The model under review builds one solid part; all positions refer to its coordinate system, in mm. Round coordinates to 2 decimals unless told otherwise and drop trailing zeros. Order: outer loops, then holes, each group sorted by start corner. A loop starts at its lowest first (then second) coordinate and runs counter-clockwise, first axis right, second up. Notation, with made-up numbers: M 2.25,-5.75 L 43.25,-5.75 A18 cw 43.25,20.25 Z; hole C -8.75,26 d2. An arc over 180 degrees is marked long. Answer as a JSON object with one key per item and string values. Group by question number.
1. Mouldability with a two-part tool opening along X and no side actions: class faces 1 (the face through (6.988, -4.115, 2.083)), 2 (the face through (0.507, 4.674, 4.365)), 3 (the face through (6.4, -3.7, 0)), 4 (the face through (12.34, 4.56, 8.71)) as released by +X, released by -X, zero draft, split by the parting line, or undercut.
2. Add section B-B on x = 11.75. State the section outline as (y, z) points, and give its area (3 significant figures).
3. Clearance check with flat-ended pins moving along their axes: P1, Ø4.5, axis at x = 6.5, y = -7.83, coming from the -Z side; P2, Ø6, axis at x = 11, y = -0.5, coming from the +Z side. State where each tip first meets the part, or that it passes through.
4. Add section A-A on z = 7.5. State the section outline as (x, y) points.
5. To check wall thickness, follow probe 1 along Y at (x, z) = (6.5, 2.6); probe 2 along Y at (x, z) = (4, 1); probe 3 along X at (y, z) = (-7.75, 4). State the ranges of each line that lie inside material, in increasing order. Write a range as [from, to].
```python
from build123d import *

# Parameters (mm, degrees)
RESSALTO_EXTRUS_O1_DEPTH = 13
ESBO_O3_R                = 3.75
CORTE_EXTRUS_O1_DEPTH    = 15
FILETE1_R                = 0.5


with BuildPart() as part:
    # Esboço2 → Ressalto-extrusão1 (new body)
    with BuildSketch(Plane(origin=(0, 0, 0), x_dir=(0, 0, -1), z_dir=(1, 0, 0))):
        Polygon((0, 5.167385512), (0, -18.032614488), (-9.609754647, 5.167385512), align=None)
    extrude(amount=RESSALTO_EXTRUS_O1_DEPTH)

    # Esboço3 → Corte-extrusão1 (cut)
    with BuildSketch(Plane(origin=(0, 0, 0), x_dir=(-1, 0, 0), z_dir=(0, 0, -1))):
        with Locations((-6.5, -7.832614488)):
            Circle(ESBO_O3_R)
    extrude(amount=-CORTE_EXTRUS_O1_DEPTH, mode=Mode.SUBTRACT)

    # Chanfro1
    # the kernel refuses this chamfer: 1, 0.765366865 mm, written as the material it takes off along each edge
    with BuildSketch(Plane(origin=(12.333333333, 4.598349918, 8.679921653), x_dir=(0.6671683756339832, -0.6671683756339838, -0.3313196600080107), z_dir=(0.7268306825413349, 0.4856527354584224, 0.485652735458423))) as chanfro1_piece_1:
        Polygon((-0.578784303, 0.323797402), (0.920087701, 0.323797402), (-0.341303398, -0.647594805), align=None)
    extrude(amount=1.33373176, mode=Mode.SUBTRACT)
    with BuildSketch(Plane(origin=(0.666666667, 4.598349918, 8.679921653), x_dir=(-0.6671683756339831, -0.6671683756339838, -0.3313196600080107), z_dir=(-0.7268306825413349, 0.48565273545842236, 0.485652735458423))) as chanfro1_piece_2:
        Polygon((-0.578784303, -0.323797402), (0.920087701, -0.323797402), (-0.341303398, 0.647594805), align=None)
    extrude(amount=1.33373176, mode=Mode.SUBTRACT)
    with BuildSketch(Plane(origin=(13, 5.167385512, 12.181437635), x_dir=(-0.9996219169112968, 0.02749587661058651, 0), z_dir=(0, 0, -1))) as chanfro1_piece_3:
        with BuildLine():
            Line((1.028673195, 0), (-0.056547155, -1.027117794))
            Line((-0.056547155, -1.027117794), (-0.076539593, -1.026567876))
            ThreePointArc((-0.076539593, -1.026567876), (-0.034129227, -0.51339783), (-0.019992438, 0.000549918))
            Line((-0.019992438, 0.000549918), (0.000549918, 0.019992438))
            ThreePointArc((0.000549918, 0.019992438), (0.514497665, 0.00585565), (1.029223113, 0.019992438))
            Line((1.029223113, 0.019992438), (1.028673195, 0))
        make_face()
    extrude(amount=14.753120623, mode=Mode.SUBTRACT)
    with BuildSketch(Plane(origin=(0, 5.167385512, 12.181437635), x_dir=(0.9996219169112968, 0.027495876610586494, 0), z_dir=(0, 0, -1))) as chanfro1_piece_4:
        with BuildLine():
            Line((1.028673195, 0), (-0.056547155, 1.027117794))
            Line((-0.056547155, 1.027117794), (-0.076539593, 1.026567876))
            ThreePointArc((-0.076539593, 1.026567876), (-0.034129227, 0.51339783), (-0.019992438, -0.000549918))
            Line((-0.019992438, -0.000549918), (0.000549918, -0.019992438))
            ThreePointArc((0.000549918, -0.019992438), (0.514497665, -0.00585565), (1.029223113, -0.019992438))
            Line((1.029223113, -0.019992438), (1.028673195, 0))
        make_face()
    extrude(amount=14.753120623, mode=Mode.SUBTRACT)
    with BuildSketch(Plane(origin=(0, -20.408539765, -0.984140473), x_dir=(-0.027495876610586358, 0.3825387462309866, -0.9235302292840447), z_dir=(0, 0.9238795325112864, 0.3826834323650908))) as chanfro1_piece_5:
        with BuildLine():
            Line((1.028673195, 0), (-0.056547155, -1.027117794))
            Line((-0.056547155, -1.027117794), (-0.076539593, -1.026567876))
            ThreePointArc((-0.076539593, -1.026567876), (-0.034129227, -0.51339783), (-0.019992438, 0.000549918))
            Line((-0.019992438, 0.000549918), (0.000549918, 0.019992438))
            ThreePointArc((0.000549918, 0.019992438), (0.514497665, 0.00585565), (1.029223113, 0.019992438))
            Line((1.029223113, 0.019992438), (1.028673195, 0))
        make_face()
    extrude(amount=30.254865023, mode=Mode.SUBTRACT)
    with BuildSketch(Plane(origin=(13, -20.408539765, -0.984140473), x_dir=(0.027495876610585605, 0.38253874623098666, -0.9235302292840448), z_dir=(0, 0.9238795325112864, 0.3826834323650908))) as chanfro1_piece_6:
        with BuildLine():
            Line((1.028673195, 0), (-0.056547155, 1.027117794))
            Line((-0.056547155, 1.027117794), (-0.076539593, 1.026567876))
            ThreePointArc((-0.076539593, 1.026567876), (-0.034129227, 0.51339783), (-0.019992438, -0.000549918))
            Line((-0.019992438, -0.000549918), (0.000549918, -0.019992438))
            ThreePointArc((0.000549918, -0.019992438), (0.514497665, -0.00585565), (1.029223113, -0.019992438))
            Line((1.029223113, -0.019992438), (1.028673195, 0))
        make_face()
    extrude(amount=30.254865023, mode=Mode.SUBTRACT)
    with BuildSketch(Plane(origin=(-2.571682988, 5.167385512, 9.609754647), x_dir=(0, 0.02749587661058651, -0.9996219169112968), z_dir=(1, 0, 0))) as chanfro1_piece_7:
        with BuildLine():
            Line((1.028673195, 0), (0.244288682, -0.742388668))
            Line((0.244288682, -0.742388668), (0.225607633, -0.749531386))
            ThreePointArc((0.225607633, -0.749531386), (0.120722331, -0.371738041), (-0.018681049, -0.007142717))
            Line((-0.018681049, -0.007142717), (0.000549918, 0.019992438))
            ThreePointArc((0.000549918, 0.019992438), (0.514497665, 0.00585565), (1.029223113, 0.019992438))
            Line((1.029223113, 0.019992438), (1.028673195, 0))
        make_face()
    extrude(amount=18.143365976, mode=Mode.SUBTRACT)

    # Filete1
    filete1_edges = [part.edges().sort_by_distance(p)[0] for p in [
        (10.25, -7.832628458, 4.22497255),
    ]]
    fillet(filete1_edges, radius=FILETE1_R)


solid = part.part
```
Recorded:
{
 "1": {"face 1": "undercut", "face 2": "released by -X", "face 3": "zero draft", "face 4": "released by +X"},
 "2": {"outline": "M -18.03,0 L 5.17,0 L 5.17,8.61 L 4.46,9.32 Z", "area": "111 mm²"},
 "3": {"P1": "passes through", "P2": "stops at z = 8.5"},
 "4": {"outline": "M 0,2.69 L 1,0.07 L 12,0.07 L 13,2.69 L 13,4.17 L 12,5.17 L 1,5.17 L 0,4.17 Z"},
 "5": {"probe 1": "y = [-4.08, 5.17]", "probe 2": "y = [-15.62, -10.63], [-5.04, 5.17]", "probe 3": "x = [0.76, 2.68], [10.32, 12.24]"}
}
